Work out the finished part from the listing and answer in its coordinate system (mm). A direction names the side the tool comes from. Give positions to 0.01 mm unless a question says otherwise; leave off trailing zeros. Loops run counter-clockwise (first coordinate to the right, second up) from the corner with the lowest first, then second, coordinate; pieces in that order, holes last. Notation, with made-up numbers: M 22,4.25 L 56,4.25 A28 cw 56,29.25 Z; hole C 47,33.25 d1. An arc over 180 degrees is marked long. Write item = value, one per line. Start each with the question number.
1. Section A-A on z = 2.25 is taken. Determine the outline of the cut face in (x, y), plus the area to 3 significant figures.
2. Section B-B on x = -27 is taken. Determine the outline of the cut face in (y, z), plus the area to 3 significant figures.
3. Flat-ended cylindrical pins translate along their axes: pin 1 Ø5.5 at (x, y) = (29.5, 14) entering from -Z; pin 2 Ø9.5 at (x, z) = (31.24, 9.42) entering from +Y. Find the tip coordinate at first contact, or state that the pin passes through.
4. Consider L1, parallel to Y at x = 26, z = 13; L2, parallel to X at y = 19, z = 14; L3, parallel to Z at x = 3.5, y = 17.75. Determine where each line is inside the solid, lowest interval first. Write a range as [from, to].
5. For faces 1 (the face through (7, 12, 20.228)), 2 (the face through (7, 21.59, 7)), determine the directions among +Z, -Z, +X, -X, +Y, -Y from which every point of the face is accessible in a straight line to the end or side of a thin tool.
6. Section C-C on z = 11 is taken. Determine the outline of the cut face in (x, y), plus the area to 3 significant figures.
7. The mould has two halves that part along X. Classify faces 3 (the face through (-39.139, 12, 8)), 4 (the face through (55.072, 12, 8)), 5 (the face through (-19.543, 1.288, 6.973)): released by +X, released by -X, zero draft, split by the parting line, or undercut.
8. Section D-D on y = 18.5 is taken. Determine the outline of the cut face in (x, z).
```python
from build123d import *

# Parameters (mm, degrees)
F0_W     = 94.210912
F0_H     = 24.106908
F1_DEPTH = 24.13
F2_T     = -2.54
F4_D     = 7.1374


with BuildPart() as f1:
    # F0 (on Front) → F1 (new body)
    with BuildSketch(Plane.XZ):
        with Locations((7.966364, 8.174181)):
            Rectangle(F0_W, F0_H)
    extrude(amount=-F1_DEPTH)

    # F2
    f2_openings = [f1.faces().sort_by_distance(p)[0] for p in [
        (7.966364, 12.065, -3.879273),
    ]]
    offset(amount=F2_T, openings=f2_openings)

    # F4 (through all)
    with Locations(Plane.XZ):
        with Locations((-22.375092, 9.144), (31.242, 9.421091)):
            Hole(F4_D / 2)


solid = f1.part
```
Verdict:
q1.outline = M -39.14,0 L 55.07,0 L 55.07,24.13 L -39.14,24.13 Z; hole M -36.6,2.54 L 52.53,2.54 L 52.53,21.59 L -36.6,21.59 Z
q1.area = 575 mm2
q2.outline = M 0,-3.88 L 2.54,-3.88 L 2.54,17.69 L 21.59,17.69 L 21.59,-3.88 L 24.13,-3.88 L 24.13,20.23 L 0,20.23 Z
q2.area = 171 mm2
q3.pin_1 = 17.69
q3.pin_2 = 24.13
q4.L1 = [0, 2.54], [21.59, 24.13]
q4.L2 = [-39.14, -36.6], [52.53, 55.07]
q4.L3 = [17.69, 20.23]
q5.face_1 = +Z, +X, -X, +Y, -Y
q5.face_2 = -Z
q6.outline = M -39.14,0 L -25.42,0 L -25.42,2.54 L -36.6,2.54 L -36.6,21.59 L -25.42,21.59 L -25.42,24.13 L -39.14,24.13 Z; M -19.33,0 L 28.04,0 L 28.04,2.54 L -19.33,2.54 Z; M -19.33,21.59 L 28.04,21.59 L 28.04,24.13 L -19.33,24.13 Z; M 34.44,0 L 55.07,0 L 55.07,24.13 L 34.44,24.13 L 34.44,21.59 L 52.53,21.59 L 52.53,2.54 L 34.44,2.54 Z
q6.area = 512 mm2
q7.face_3 = released by -X
q7.face_4 = released by +X
q7.face_5 = undercut
q8.outline = M -39.14,-3.88 L -36.6,-3.88 L -36.6,17.69 L 52.53,17.69 L 52.53,-3.88 L 55.07,-3.88 L 55.07,20.23 L -39.14,20.23 Z
